```python
from build123d import *

# Parameters (mm, degrees)
SKETCH1_R           = 1.5875
SKETCH1_R_2         = 6.35
SKETCH1_W           = 25.4
SKETCH1_H           = 6.35
SKETCH1_W_2         = 6.35
SKETCH1_H_2         = 25.4
BOSS_EXTRUDE1_DEPTH = 6.35


with BuildPart() as part:
    # Sketch1 → Boss-Extrude1 (new body)
    with BuildSketch(Plane(origin=(0, 0, 0), x_dir=(1, 0, 0), z_dir=(0, 1, 0))):
        with BuildLine():
            Line((-158.372209236, 3.874169231), (-259.972209236, 3.874169231))
            Line((-259.972209236, 3.874169231), (-259.972209236, 41.974169231))
            ThreePointArc((-259.972209236, 41.974169231), (-248.8129776, 68.914937594), (-221.872209236, 80.074169231))
            Line((-221.872209236, 80.074169231), (82.172209236, 80.074169231))
            ThreePointArc((82.172209236, 80.074169231), (179.256365551, 59.708562917), (259.972209236, 2.045369231))
            Line((259.972209236, 2.045369231), (234.572209236, 2.045369231))
            Line((234.572209236, 2.045369231), (234.572209236, -4.304630769))
            Line((234.572209236, -4.304630769), (259.972209236, -4.304630769))
            ThreePointArc((259.972209236, -4.304630769), (179.256365551, -61.967824455), (82.172209236, -82.333430769))
            Line((82.172209236, -82.333430769), (-221.872209236, -82.333430769))
            ThreePointArc((-221.872209236, -82.333430769), (-248.8129776, -71.174199132), (-259.972209236, -44.233430769))
            Line((-259.972209236, -44.233430769), (-259.972209236, -6.133430769))
            Line((-259.972209236, -6.133430769), (-158.372209236, -6.133430769))
            Line((-158.372209236, -6.133430769), (-147.882694507, -6.133430769))
            ThreePointArc((-147.882694507, -6.133430769), (-145.777792064, -1.129630769), (-147.882694507, 3.874169231))
            Line((-147.882694507, 3.874169231), (-158.372209236, 3.874169231))
        make_face()
        with Locations(Location((-190.877790764, -39.229630769, 0), (0, 0, 270))):
            Circle(SKETCH1_R, mode=Mode.SUBTRACT)
        with Locations(Location((-114.677790764, -39.229630769, 0), (0, 0, 270))):
            Circle(SKETCH1_R, mode=Mode.SUBTRACT)
        with Locations(Location((-114.677790764, 36.970369231, 0), (0, 0, 270))):
            Circle(SKETCH1_R, mode=Mode.SUBTRACT)
        with Locations(Location((-190.877790764, 36.970369231, 0), (0, 0, 270))):
            Circle(SKETCH1_R, mode=Mode.SUBTRACT)
        with Locations(Location((120.272209236, -1.129630769, 0), (0, 0, 270))):
            Circle(SKETCH1_R, mode=Mode.SUBTRACT)
        with Locations(Location((171.072209236, -1.129630769, 0), (0, 0, 270))):
            Circle(SKETCH1_R, mode=Mode.SUBTRACT)
        with Locations(Location((221.872209236, -1.129630769, 0), (0, 0, 270))):
            Circle(SKETCH1_R, mode=Mode.SUBTRACT)
        with Locations(Location((78.997209236, 14.745369231, 0), (0, 0, 270))):
            Circle(SKETCH1_R, mode=Mode.SUBTRACT)
        with Locations(Location((78.997209236, 66.459769231, 0), (0, 0, 270))):
            Circle(SKETCH1_R, mode=Mode.SUBTRACT)
        with Locations(Location((-21.766377903, 47.368819725, 0), (0, 0, 270))):
            Circle(SKETCH1_R_2, mode=Mode.SUBTRACT)
        with Locations(Location((-221.872209236, 73.724169231, 0), (0, 0, 270))):
            Circle(SKETCH1_R, mode=Mode.SUBTRACT)
        with Locations(Location((-69.85, 73.724169231, 0), (0, 0, 270))):
            Circle(SKETCH1_R, mode=Mode.SUBTRACT)
        with Locations((94.872209236, -1.129630769)):
            Rectangle(SKETCH1_W, SKETCH1_H, mode=Mode.SUBTRACT)
        with Locations((145.672209236, -1.129630769)):
            Rectangle(SKETCH1_W, SKETCH1_H, mode=Mode.SUBTRACT)
        with Locations((196.472209236, -1.129630769)):
            Rectangle(SKETCH1_W, SKETCH1_H, mode=Mode.SUBTRACT)
        with Locations((78.997209236, 40.145369231)):
            Rectangle(SKETCH1_W_2, SKETCH1_H_2, mode=Mode.SUBTRACT)
        Polygon((-221.872209236, 67.374169231), (-218.697209236, 67.374169231), (-218.697209236, 54.674169231), (-225.047209236, 54.674169231), (-225.047209236, 67.374169231), align=None, mode=Mode.SUBTRACT)
        Polygon((-69.85, 67.374169231), (-66.675, 67.374169231), (-66.675, 54.674169231), (-73.025, 54.674169231), (-73.025, 67.374169231), align=None, mode=Mode.SUBTRACT)
    extrude(amount=BOSS_EXTRUDE1_DEPTH)


solid = part.part
```
Here's how the part is built. I have some questions about the finished solid (model axes, mm). Round coordinates to 2 decimals unless told otherwise and drop trailing zeros. Loops run counter-clockwise (first coordinate to the right, second up) from the corner with the lowest first, then second, coordinate; pieces in that order, holes last.
1. Suppose I cut it at C-C, the plane z = 22. Please give me the cut outline in (x, y), and give its area (3 significant figures).
Answers:
outline: (-259.97, 0) - (241.89, 0) - (241.89, 6.35) - (-259.97, 6.35) - close
area: 3,190 mm2
2. Will these pins go through, and if not, where does the flat tip stop? pin 1 (1 mm diameter, centred on y = 3.5, z = -12, fed in from +X); pin 2 (1.9 mm diameter, centred on y = 4, z = -63.5, fed in from -X); pin 3 (1.9 mm diameter, centred on y = 2.5, z = -45, fed in from -X).
Answers:
pin 1: stops at x = 250.79
pin 2: stops at x = -253.94
pin 3: stops at x = -259.92
3. Suppose I cut it at A-A, the plane x = -201. Please give me the cut outline in (y, z), and give its area (3 significant figures).
Answers:
outline: (0, -80.07) - (6.35, -80.07) - (6.35, -3.87) - (0, -3.87) - close; (0, 6.13) - (6.35, 6.13) - (6.35, 82.33) - (0, 82.33) - close
area: 968 mm2
4. If I drill on probe 1 along Z at (x, y) = (-221.5, 4.5); probe 2 along X at (y, z) = (4.75, -42); probe 3 along Z at (x, y) = (-193, 1.5), over which ranges is the centre line in solid material (lowest first)?
Answers:
probe 1: z = -80.07 to -75.27, -72.18 to -67.37, -54.67 to -3.87, 6.13 to 82.33
probe 2: x = -259.97 to -25.16, -18.38 to 75.82, 82.17 to 212.35
probe 3: z = -80.07 to -3.87, 6.13 to 82.33
5. Suppose I cut it at B-B, the plane y = 4.5. Give the number of separate pieces and of enclosed holes in the cut face, and give its area (3 significant figures).
Answers:
separate pieces: 1
enclosed holes: 18
area: 72,900 mm2
6. Thinking about a two-plate mould opening in Z: for faces 1 (the face through (4, 0, 0)), 2 (the face through (-248.515, 3.131, 71.469)), 3 (the face through (-24.198, 3.131, -41.503)), 4 (the face through (-249.108, 3.131, -68.617)), which applies, released by +Z, released by -Z, zero draft, split by the parting line, or undercut?
Answers:
face 1: zero draft
face 2: released by +Z
face 3: undercut
face 4: released by -Z
